from build123d import *

# Parameters (mm, degrees)
SKETCH3_R          = 5.5
CUT_EXTRUDE1_DEPTH = 132.030215122
SKETCH4_R          = 5.481177192
CUT_EXTRUDE2_DEPTH = 126.624122086


with BuildPart() as part:
    # Sketch2 → Revolve1 (revolve)
    with BuildSketch(Plane.XY):
        Polygon((0, 0), (0, 86.995), (5.08, 86.995), (8.781317037, 79.0575), (10.903682963, 79.0575), (14.605, 86.995), (19.685, 86.995), (19.685, 38.1), (45.085, 38.1), (45.085, 0), align=None)
    revolve(axis=Axis((45.085, 0, 0), (-1, 0, 0)))

    # Sketch3 → Cut-Extrude1 (cut, through all)
    with BuildSketch(Plane(origin=(45.085, 0, 0), x_dir=(0, 0, -1), z_dir=(1, 0, 0))):
        with Locations(Location((0, 0, 0), (0, 0, 90))):
            Circle(SKETCH3_R)
    extrude(amount=-CUT_EXTRUDE1_DEPTH, mode=Mode.SUBTRACT)

    # Sketch4 → Cut-Extrude2 (cut, through all)
    with BuildSketch(Plane(origin=(19.685, 0, 0), x_dir=(0, 0, -1), z_dir=(1, 0, 0))):
        with Locations(Location((0, 61.039888565, 0), (0, 0, 90))):
            Circle(SKETCH4_R)
        with Locations(Location((52.862094142, -30.519944283, 0), (0, 0, 90))):
            Circle(SKETCH4_R)
        with Locations(Location((-52.862094142, -30.519944283, 0), (0, 0, 90))):
            Circle(SKETCH4_R)
    extrude(amount=-CUT_EXTRUDE2_DEPTH, mode=Mode.SUBTRACT)


solid = part.part
Design review of the part built by this model. Coordinates are the model's own, in mm. A direction names the side the tool comes from. Give positions to 0.01 mm unless a question says otherwise; leave off trailing zeros. Loops run counter-clockwise (first coordinate to the right, second up) from the corner with the lowest first, then second, coordinate; pieces in that order, holes last. Notation, with made-up numbers: (74.5, -21.5) - (79.5, -21.5) arc R25 ccw to (79.5, 6.5) - close; hole circle Ø1 at (83.5, -4.75). An arc over 180 degrees is marked (long way). Write item = value, one per line.
1) Take a section at A-A on z = 0. State the section outline as (x, y) points (1 decimal), and give its area (3 significant figures).
Result sheet:
outline = (0, -87) - (5.1, -87) - (8.8, -79.1) - (10.9, -79.1) - (14.6, -87) - (19.7, -87) - (19.7, -38.1) - (45.1, -38.1) - (45.1, -5.5) - (0, -5.5) - close; (0, 5.5) - (45.1, 5.5) - (45.1, 38.1) - (19.7, 38.1) - (19.7, 55.6) - (0, 55.6) - close; (0, 66.5) - (19.7, 66.5) - (19.7, 87) - (14.6, 87) - (10.9, 79.1) - (8.8, 79.1) - (5.1, 87) - (0, 87) - close
area = 4,560 mm2
2) Clearance check with flat-ended pins moving along their axes: pin 1 Ø2 at (x, z) = (29, 16.5) entering from -Y; pin 2 Ø12 at (x, z) = (21.5, 5) entering from -Y (3 decimals); pin 3 Ø17.5 at (y, z) = (61.04, 0) entering from +X (3 decimals); pin 4 Ø12 at (x, y) = (22, 23) entering from +Z. State where each tip first meets the part, or that it passes through.
Result sheet:
pin_1 = -34.8
pin_2 = -86.995
pin_3 = 19.685
pin_4 = 85.22
3) Take a section at B-B on y = 0. State the section outline as (x, z) points (1 decimal), and give its area (3 significant figures).
Result sheet:
outline = (0, -87) - (5.1, -87) - (8.8, -79.1) - (10.9, -79.1) - (14.6, -87) - (19.7, -87) - (19.7, -38.1) - (45.1, -38.1) - (45.1, -5.5) - (0, -5.5) - close; (0, 5.5) - (45.1, 5.5) - (45.1, 38.1) - (19.7, 38.1) - (19.7, 87) - (14.6, 87) - (10.9, 79.1) - (8.8, 79.1) - (5.1, 87) - (0, 87) - close
area = 4,770 mm2
4) Take a section at C-C on x = 30. State the section outline as (y, z) points, and give its area (3 significant figures).
Result sheet:
outline = circle Ø76.2 at (0, 0); hole circle Ø11 at (0, 0)
area = 4,470 mm2
5) Draft analysis for pull direction Y (two halves, no side actions). For faces 4 (the face through (45.085, 8, -1)), 5 (the face through (22.86, -1.19, -5.37)), 6 (the face through (17.181, -18.859, 84.926)), state which applies: +Y half, -Y half, draft (parallel to the pull), parting line (faces both ways), or undercut.
Result sheet:
face_4 = draft
face_5 = undercut
face_6 = parting line
6) Tool access review of faces 1 (the face through (11.135, -17.246, 77.662)), 2 (the face through (9.98, -31.71, 47.51)), 3 (the face through (32.563, -30.235, 23.183)): name each direction out of +Z, -Z, +X, -X, +Y, -Y from which nothing blocks a thin tool from reaching the whole face with its end or side.
Result sheet:
face_1 = none
face_2 = +X, -X
face_3 = +X
7) To check wall thickness, follow line 1 (Z direction, x = 25, y = 0); line 2 (Y direction, x = 19, z = -3); line 3 (X direction, y = 43.5, z = -28) (3 decimals). State the ranges of each line that lie inside material, in increasing order.
Result sheet:
line_1 = -38.1 to -5.5, 5.5 to 38.1
line_2 = -86.94 to -4.61, 4.61 to 56.45, 65.63 to 86.94
line_3 = 0 to 19.685
